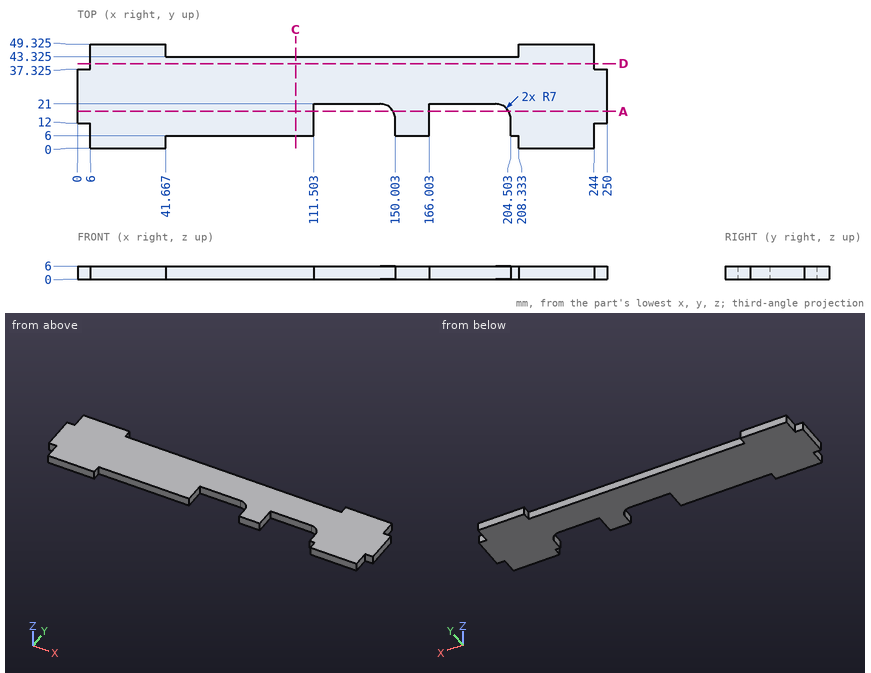
Design review of the part shown in the three views and the two pictorial views. Dimensions are in mm from the part's minimum x, y and z. Coordinates: 2 decimals unless noted, no trailing zeros. Loops run counter-clockwise (first coordinate to the right, second up) from the corner with the lowest first, then second, coordinate; pieces in that order, holes last. Notation, with made-up numbers: (-21, 77) -> (0, 77) arc R9 cw to (0, 86) -> close; hole circle Ø2 at (81.25, -1.5). An arc over 180 degrees is marked (long way). Answer as CSV lines item,"result".
Item 1: For L1, parallel to X at y = 13.5, z = 4.05; L2, parallel to X at y = 19.5, z = 2.1 (1 decimal); L3, parallel to Y at x = 95.5, z = 1.8 (1 decimal), list the stretches that pass through material, from the lowest coordinate up.
Results below:
L1,"x = 0 to 111.5, 150 to 166, 204.5 to 250"
L2,"x = 0 to 111.5, 147.3 to 166, 201.8 to 250"
L3,"y = 6 to 43.3"
Item 2: Take a section at D-D, the plane y = 40. State the section outline as (x, z) points, and give its area (3 significant figures).
Results below:
outline,"(6, 0) -> (244, 0) -> (244, 6) -> (6, 6) -> close"
area,"1,430 mm2"
Item 3: Take a section at A-A, the plane y = 17.5. State the section outline as (x, z) points (1 decimal), and give its area (3 significant figures).
Results below:
outline,"(0, 0) -> (111.5, 0) -> (111.5, 6) -> (0, 6) -> close; (149.1, 0) -> (166, 0) -> (166, 6) -> (149.1, 6) -> close; (203.6, 0) -> (250, 0) -> (250, 6) -> (203.6, 6) -> close"
area,"1,050 mm2"
Item 4: Take a section at C-C, the plane x = 103. State the section outline as (y, z) points (1 decimal), and give its area (3 significant figures).
Results below:
outline,"(6, 0) -> (43.3, 0) -> (43.3, 6) -> (6, 6) -> close"
area,"224 mm2"
Item 5: Insertion check: pin 1 (1.8 mm diameter, centred on x = 177.5, z = 3, fed in from -Y); pin 2 (3 mm diameter, centred on x = 247, z = 3.5, fed in from +Y) (3 decimals); pin 3 (1.8 mm diameter, centred on y = 42.5, z = 4, fed in from -X). Each pin has a flat end and moves straight along its axis. Give the tip position at first contact, or say it passes through.
Results below:
pin 1,"stops at y = 21"
pin 2,"stops at y = 37.325"
pin 3,"stops at x = 6"
